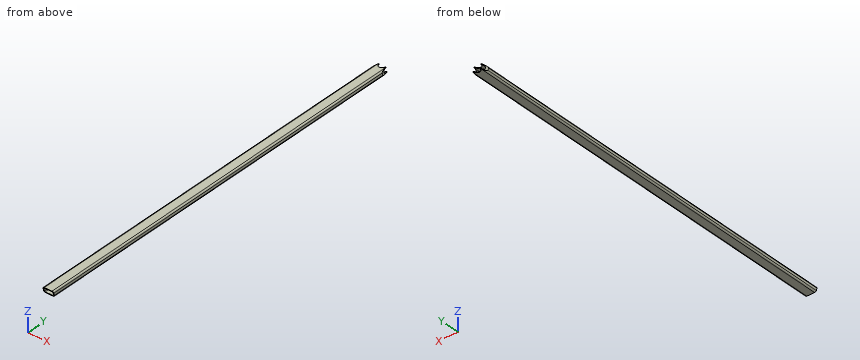
```python
from build123d import *

# Parameters (mm, degrees)
EXTRUDE_1_DEPTH     = 1130
CUT_EXTRUDE_1_DEPTH = 40


with BuildPart() as part:
    # Эскиз1 → Вытянуть-Тонкостенный1 (new body)
    with BuildSketch(Plane(origin=(0, 0, 0), x_dir=(1, 0, 0), z_dir=(0, 1, 0))):
        with BuildLine():
            Line((-11, 7.5), (11, 7.5))
            ThreePointArc((11, 7.5), (13.828427125, 6.328427125), (15, 3.5))
            Line((15, 3.5), (15, -3.5))
            ThreePointArc((15, -3.5), (13.828427125, -6.328427125), (11, -7.5))
            Line((11, -7.5), (-11, -7.5))
            ThreePointArc((-11, -7.5), (-13.828427125, -6.328427125), (-15, -3.5))
            Line((-15, -3.5), (-15, 3.5))
            ThreePointArc((-15, 3.5), (-13.828427125, 6.328427125), (-11, 7.5))
        make_face()
        with BuildLine():
            Line((-11, 5.5), (11, 5.5))
            ThreePointArc((11, 5.5), (12.414213562, 4.914213562), (13, 3.5))
            Line((13, 3.5), (13, -3.5))
            ThreePointArc((13, -3.5), (12.414213562, -4.914213562), (11, -5.5))
            Line((11, -5.5), (-11, -5.5))
            ThreePointArc((-11, -5.5), (-12.414213562, -4.914213562), (-13, -3.5))
            Line((-13, -3.5), (-13, 3.5))
            ThreePointArc((-13, 3.5), (-12.414213562, 4.914213562), (-11, 5.5))
        make_face(mode=Mode.SUBTRACT)
    extrude(amount=EXTRUDE_1_DEPTH)

    # Surface Cut 2
    split(bisect_by=Plane(origin=(0, 1052.429353138, 281.997595264), x_dir=(-1, 0, 0), z_dir=(0, 0.9659258262890681, 0.25881904510252135)), keep=Keep.BOTTOM)

    # Эскиз4 → Вырез-Вытянуть1 (cut)
    with BuildSketch(Plane(origin=(0, 77.570646862, -289.497595264), x_dir=(-1, 0, 0), z_dir=(0, 0.25881904510252135, -0.9659258262890681))):
        with BuildLine():
            Line((-9, 1089.555040868), (-10, 1089.555040868))
            Line((-10, 1089.555040868), (-20, 1052.234532793))
            Line((-20, 1052.234532793), (-20, 1094.555040868))
            Line((-20, 1094.555040868), (20, 1094.555040868))
            Line((20, 1094.555040868), (20, 1052.234532793))
            Line((20, 1052.234532793), (10, 1089.555040868))
            Line((10, 1089.555040868), (9, 1089.555040868))
            ThreePointArc((9, 1089.555040868), (0, 1080.555040868), (-9, 1089.555040868))
        make_face()
    extrude(amount=-CUT_EXTRUDE_1_DEPTH, mode=Mode.SUBTRACT)

    # Surface Cut 3
    split(bisect_by=Plane(origin=(0, 1.875, 0.502404736), x_dir=(1, 0, 0), z_dir=(0, 0.9659258262890691, 0.25881904510251796)), keep=Keep.TOP)


solid = part.part
```
Input: part model. Units: mm. Frame: model coordinates. Coordinates: 2 decimals unless noted, no trailing zeros. Loops run counter-clockwise (first coordinate to the right, second up) from the corner with the lowest first, then second, coordinate; pieces in that order, holes last. Notation, with made-up numbers: (38, 18) -> (95, 18) arc R34 cw to (95, 49) -> close; hole circle Ø11 at (-22.75, 88.25). An arc over 180 degrees is marked (long way). Use a Markdown table: item, result.
1) Material intervals for line 1 along X through (y, z) = (306, -2.5); line 2 along Z through (x, y) = (4, 853); line 3 along X through (y, z) = (999, -4.25), sorted ascending. Write a range as from..to.
Results found:
| item | result |
|---|---|
| line 1 | x = -15..-13, 13..15 |
| line 2 | z = -7.5..-5.5, 5.5..7.5 |
| line 3 | x = -14.93..-12.85, 12.85..14.93 |
2) Cut plane A-A (y = 918). Return the cut outline in (x, z).
Results found:
| item | result |
|---|---|
| outline | (-15, -3.5) arc R4 ccw to (-11, -7.5) -> (11, -7.5) arc R4 ccw to (15, -3.5) -> (15, 3.5) arc R4 ccw to (11, 7.5) -> (-11, 7.5) arc R4 ccw to (-15, 3.5) -> close; hole (-13, -3.5) arc R2 ccw to (-11, -5.5) -> (11, -5.5) arc R2 ccw to (13, -3.5) -> (13, 3.5) arc R2 ccw to (11, 5.5) -> (-11, 5.5) arc R2 ccw to (-13, 3.5) -> close |
3) Cut plane B-B (x = 1). Return the cut outline in (y, z).
Results found:
| item | result |
|---|---|
| outline | (0, 7.5) -> (0.54, 5.5) -> (1117.26, 5.5) -> (1116.72, 7.5) -> close; (3.48, -5.5) -> (4.02, -7.5) -> (1120.74, -7.5) -> (1120.2, -5.5) -> close |
4) Contact query for a flat-ended pin moving along its axis: pin 1 (6 mm diameter, centred on x = 5.5, z = -5, fed in from -Y). Output: stop coordinate, or through.
Results found:
| item | result |
|---|---|
| pin 1 | stops at y = 3.48 |
